from build123d import *

# Parameters (mm, degrees)
BOSS_EXTRUDE1_DEPTH = 6.3
SKETCH2_W           = 9.11
SKETCH2_H           = 5.95
BOSS_EXTRUDE2_DEPTH = 15
FILLET1_R           = 1.4
SKETCH4_R           = 2.845
BOSS_EXTRUDE3_DEPTH = 6.74
SKETCH5_R           = 1.6
BOSS_EXTRUDE4_DEPTH = 2


with BuildPart() as part:
    # Sketch1 → Boss-Extrude1 (new body)
    with BuildSketch(Plane(origin=(0, 0, 0), x_dir=(1, 0, 0), z_dir=(0, 1, 0))):
        Polygon((-3.42, 0), (-2.68, -0.9), (2.68, -0.9), (3.42, 0), (3.42, 0.9), (-3.42, 0.9), align=None)
    extrude(amount=BOSS_EXTRUDE1_DEPTH)

    # Sketch2 → Boss-Extrude2 (add)
    with BuildSketch(Plane(origin=(0, 6.3, 0), x_dir=(1, 0, 0), z_dir=(0, 1, 0))):
        Rectangle(SKETCH2_W, SKETCH2_H)
    extrude(amount=BOSS_EXTRUDE2_DEPTH)

    # Fillet1
    fillet1_edges = [part.edges().sort_by_distance(p)[0] for p in [
        (4.555, 13.8, 2.975),
        (4.555, 13.8, -2.975),
        (-4.555, 13.8, -2.975),
        (-4.555, 13.8, 2.975),
    ]]
    fillet(fillet1_edges, radius=FILLET1_R)

    # Sketch4 → Boss-Extrude3 (add)
    with BuildSketch(Plane(origin=(0, 21.3, 0), x_dir=(1, 0, 0), z_dir=(0, 1, 0))):
        with Locations(Location((0, 0, 0), (0, 0, 270))):
            Circle(SKETCH4_R)
    extrude(amount=BOSS_EXTRUDE3_DEPTH)

    # Sketch5 → Boss-Extrude4 (add)
    with BuildSketch(Plane(origin=(0, 28.04, 0), x_dir=(1, 0, 0), z_dir=(0, 1, 0))):
        with Locations(Location((0, 0, 0), (0, 0, 270))):
            Circle(SKETCH5_R)
    extrude(amount=BOSS_EXTRUDE4_DEPTH)


solid = part.part
CAD build for the part. Positions are in the model's coordinates, mm. A direction names the side the tool comes from. Coordinates: 2 decimals unless noted, no trailing zeros. Order: outer loops, then holes, each group sorted by start corner. A loop starts at its lowest first (then second) coordinate and runs counter-clockwise, first axis right, second up. Notation, with made-up numbers: (-24.5, 66) -> (-14.5, 66) arc R25 cw to (-14.5, 92) -> close; hole circle Ø1 at (82, 65.25). An arc over 180 degrees is marked (long way). Answer in a Markdown table with one row per item.
1) Band-saw the part on A-A (x = 0). List the corners of the cut face in (y, z) (3 decimals).
Check values:
| item | result |
|---|---|
| outline | (0, -0.9) -> (6.3, -0.9) -> (6.3, -2.975) -> (21.3, -2.975) -> (21.3, -2.845) -> (28.04, -2.845) -> (28.04, -1.6) -> (30.04, -1.6) -> (30.04, 1.6) -> (28.04, 1.6) -> (28.04, 2.845) -> (21.3, 2.845) -> (21.3, 2.975) -> (6.3, 2.975) -> (6.3, 0.9) -> (0, 0.9) -> close |
2) Drill centre lines: line 1 (Z direction, x = -1, y = 6); line 2 (Y direction, x = -3.25, z = -0.35); line 3 (Y direction, x = 0.5, z = 2.35). Where is each one in solid material? Low to high.
Check values:
| item | result |
|---|---|
| line 1 | -0.9 to 0.9 |
| line 2 | 0 to 21.3 |
| line 3 | 6.3 to 28.04 |
3) Which spindle directions (+Z, -Z, +X, -X, +Y, -Y) get a long thin tool onto all of the face, cutting with end or side? Do faces 1 (the face through (0, 3, 0.9)), 2 (the face through (3.04, 3.11, 0.46)), 3 (the face through (3.42, 3.1, -0.4)), 4 (the face through (-0.97, 29.03, -1.27)). Say none if no direction does.
Check values:
| item | result |
|---|---|
| face 1 | +Z, +X, -X, -Y |
| face 2 | +Z, +X, -Y |
| face 3 | +Z, -Z, +X, -Y |
| face 4 | +Y |
4) Band-saw the part on D-D (z = -2.1). List the corners of the cut face in (x, y), and give its area (3 significant figures).
Check values:
| item | result |
|---|---|
| outline | (-4.45, 6.3) -> (4.45, 6.3) -> (4.45, 21.3) -> (1.92, 21.3) -> (1.92, 28.04) -> (-1.92, 28.04) -> (-1.92, 21.3) -> (-4.45, 21.3) -> close |
| area | 159 mm2 |
5) Flat gauge pins, fed straight in: P1, Ø0.7, axis at y = 3, z = -0.5, coming from the +X side; P2, Ø1.9, axis at x = 0, y = 4, coming from the -Z side. Where does each tip first touch, or does it go through?
Check values:
| item | result |
|---|---|
| P1 | x = 3.42 |
| P2 | z = -0.9 |
6) Band-saw the part on C-C (y = 24). List the corners of the cut face in (x, z) (3 decimals).
Check values:
| item | result |
|---|---|
| outline | circle Ø5.69 at (0, 0) |
7) Band-saw the part on B-B (z = 0.45). List the corners of the cut face in (x, y) (3 decimals).
Check values:
| item | result |
|---|---|
| outline | (-4.555, 6.3) -> (-3.05, 6.3) -> (-3.05, 0) -> (3.05, 0) -> (3.05, 6.3) -> (4.555, 6.3) -> (4.555, 21.3) -> (2.809, 21.3) -> (2.809, 28.04) -> (1.535, 28.04) -> (1.535, 30.04) -> (-1.535, 30.04) -> (-1.535, 28.04) -> (-2.809, 28.04) -> (-2.809, 21.3) -> (-4.555, 21.3) -> close |
